Work out the finished part from the listing and answer in its coordinate system (mm). A direction names the side the tool comes from. Coordinates: 2 decimals unless noted, no trailing zeros. Write each loop counter-clockwise with the first axis right and the second up, starting at its lowest first coordinate (ties: lowest second). Pieces come first, ordered by that corner, then holes. Notation, with made-up numbers: (-35, -4.5) - (2, -4.5) arc R34 ccw to (2, 31.5) - close; hole circle Ø4 at (14, 52). An arc over 180 degrees is marked (long way). Use one line per item in the form item = value. Start each with the question number.
Item 1: Consider probe 1 along X at (y, z) = (0.5, 2.75) (3 decimals); probe 2 along Z at (x, y) = (-8.5, 0.45) (3 decimals). Determine where each line is inside the solid, lowest interval first.
Item 2: Given pin 1 (3 mm diameter, centred on x = -2.5, z = -7, fed in from -Y), flat-ended and moving along its own axis, determine where the tip first touches the part or whether it passes through.
Item 3: Determine the mould class of faces 3 (the flat face through (-9, 0, 0)), 4 (the cylindrical face through (-9.997, 0.507, -9.979)), 5 (the flat face through (-0.1, 0.5, 8.825)), 6 (the flat face through (10.325, 0.5, 0.1)) for opening direction X: released by +X, released by -X, zero draft, split by the parting line, or undercut.
Item 4: A cutting plane is placed at A-A (z = 0.5). Write down the section's boundary in (x, y) (3 decimals).
Item 5: For faces 1 (the cylindrical face through (9.979, 0.507, 9.997)), 2 (the cylindrical face through (8.479, 0.493, -8.497)), determine the directions among +Z, -Z, +X, -X, +Y, -Y from which every point of the face is accessible in a straight line to the end or side of a thin tool.
Item 6: A cutting plane is placed at C-C (y = 0.6). Write down the section's boundary in (x, z) (3 decimals), then the cut area to 3 significant figures.
Item 7: A cutting plane is placed at B-B (x = -3.75). Write down the section's boundary in (y, z) (3 decimals).
from build123d import *

# Parameters (mm, degrees)
SKETCH1_W           = 20.65
SKETCH1_H           = 20.65
SKETCH1_W_2         = 17.65
SKETCH1_H_2         = 17.65
BOSS_EXTRUDE1_DEPTH = 1
FILLET1_R           = 1.15


with BuildPart() as part:
    # Sketch1 → Boss-Extrude1 (new body)
    # profile 1 of 5: a face of its own
    with BuildSketch(Plane(origin=(0, 0, 0), x_dir=(1, 0, 0), z_dir=(0, 1, 0))):
        Rectangle(SKETCH1_W, SKETCH1_H)
        Rectangle(SKETCH1_W_2, SKETCH1_H_2, mode=Mode.SUBTRACT)
    # profile 2 of 5: a face of its own
    with BuildSketch(Plane(origin=(0, 0, 0), x_dir=(1, 0, 0), z_dir=(0, 1, 0))):
        with BuildLine():
            Line((-8.825, -7.675), (-8.825, -8.825))
            Line((-8.825, -8.825), (-7.675, -8.825))
            ThreePointArc((-7.675, -8.825), (-8.488172798, -8.488172798), (-8.825, -7.675))
        make_face()
    # profile 3 of 5: a face of its own
    with BuildSketch(Plane(origin=(0, 0, 0), x_dir=(1, 0, 0), z_dir=(0, 1, 0))):
        with BuildLine():
            Line((-8.825, 8.825), (-8.825, 7.675))
            ThreePointArc((-8.825, 7.675), (-8.488172798, 8.488172798), (-7.675, 8.825))
            Line((-7.675, 8.825), (-8.825, 8.825))
        make_face()
    # profile 4 of 5: a face of its own
    with BuildSketch(Plane(origin=(0, 0, 0), x_dir=(1, 0, 0), z_dir=(0, 1, 0))):
        with BuildLine():
            ThreePointArc((7.675, 8.825), (8.488172798, 8.488172798), (8.825, 7.675))
            Line((8.825, 7.675), (8.825, 8.825))
            Line((8.825, 8.825), (7.675, 8.825))
        make_face()
    # profile 5 of 5: a face of its own
    with BuildSketch(Plane(origin=(0, 0, 0), x_dir=(1, 0, 0), z_dir=(0, 1, 0))):
        with BuildLine():
            ThreePointArc((8.825, -7.675), (8.488172798, -8.488172798), (7.675, -8.825))
            Line((7.675, -8.825), (8.825, -8.825))
            Line((8.825, -8.825), (8.825, -7.675))
        make_face()
    extrude(amount=BOSS_EXTRUDE1_DEPTH)

    # Fillet1
    fillet1_edges = [part.edges().sort_by_distance(p)[0] for p in [
        (-10.325, 0.5, 10.325),
        (-10.325, 0.5, -10.325),
        (10.325, 0.5, -10.325),
        (10.325, 0.5, 10.325),
    ]]
    fillet(fillet1_edges, radius=FILLET1_R)


solid = part.part
Answer:
q1.probe_1 = -10.325 to -8.825, 8.825 to 10.325
q1.probe_2 = -10.325 to -8.476, 8.476 to 10.325
q2.pin_1 = through
q3.face_3 = zero draft
q3.face_4 = released by -X
q3.face_5 = undercut
q3.face_6 = released by +X
q4.outline = (-10.325, 0) - (-8.825, 0) - (-8.825, 1) - (-10.325, 1) - close; (8.825, 0) - (10.325, 0) - (10.325, 1) - (8.825, 1) - close
q5.face_1 = +Z, +X, +Y, -Y
q5.face_2 = +Y, -Y
q6.outline = (-10.325, -9.175) arc R1.15 ccw to (-9.175, -10.325) - (9.175, -10.325) arc R1.15 ccw to (10.325, -9.175) - (10.325, 9.175) arc R1.15 ccw to (9.175, 10.325) - (-9.175, 10.325) arc R1.15 ccw to (-10.325, 9.175) - close; hole (-8.825, -7.675) arc R1.15 ccw to (-7.675, -8.825) - (7.675, -8.825) arc R1.15 ccw to (8.825, -7.675) - (8.825, 7.675) arc R1.15 ccw to (7.675, 8.825) - (-7.675, 8.825) arc R1.15 ccw to (-8.825, 7.675) - close
q6.area = 115 mm²
q7.outline = (0, -10.325) - (1, -10.325) - (1, -8.825) - (0, -8.825) - close; (0, 8.825) - (1, 8.825) - (1, 10.325) - (0, 10.325) - close
